```python
from build123d import *

# Parameters (mm, degrees)
F1_DEPTH = 190
F0_W     = 80
F0_H     = 30.028
F0_W_2   = 35.56
F0_H_2   = 17.78
F0_H_3   = 9.652
F0_W_3   = 2.22
F2_DEPTH = 5


with BuildPart() as f1:
    # F0 (on Front) → F1 (new body)
    with BuildSketch(Plane.XZ):
        Polygon((45, 30), (45, 35), (-40, 35), (-40, 30.452), (-40, 30), (40, 30), align=None)
        Polygon((-40, 30.452), (-40, 35), (-45, 35), (-45, -30), (-40, -30), (-40, -20.348), (-40, -19.078), (-40, -1.298), (-40, -0.028), (-40, 30), align=None)
        Polygon((45, -30), (45, 30), (40, 30), (40, -0.028), (40, -1.298), (40, -19.078), (40, -20.348), (40, -30), align=None)
        Polygon((45, -35), (45, -30), (40, -30), (4.44, -30), (2.22, -30), (-2.22, -30), (-4.44, -30), (-40, -30), (-45, -30), (-45, -35), align=None)
        Polygon((40, -1.298), (40, -0.028), (-40, -0.028), (-40, -1.298), (-4.44, -1.298), (-2.22, -1.298), (2.22, -1.298), (4.44, -1.298), align=None)
        Polygon((4.44, -20.348), (40, -20.348), (40, -19.078), (4.44, -19.078), (2.22, -19.078), (2.22, -20.348), align=None)
        Polygon((-40, -19.078), (-40, -20.348), (-4.44, -20.348), (-2.22, -20.348), (-2.22, -19.078), (-4.44, -19.078), align=None)
        Polygon((-2.22, -30), (2.22, -30), (2.22, -20.348), (2.22, -19.078), (2.22, -1.298), (-2.22, -1.298), (-2.22, -19.078), (-2.22, -20.348), align=None)
    extrude(amount=F1_DEPTH)

    # F0 (on Front) → F2 (join)
    with BuildSketch(Plane.XZ):
        with Locations((0, 14.986)):
            Rectangle(F0_W, F0_H)
        with Locations((-22.22, -10.188)):
            Rectangle(F0_W_2, F0_H_2)
        with Locations((22.22, -10.188)):
            Rectangle(F0_W_2, F0_H_2)
        with Locations((22.22, -25.174)):
            Rectangle(F0_W_2, F0_H_3)
        with Locations((-22.22, -25.174)):
            Rectangle(F0_W_2, F0_H_3)
        with Locations((-3.33, -10.188)):
            Rectangle(F0_W_3, F0_H_2)
        with Locations((-3.33, -25.174)):
            Rectangle(F0_W_3, F0_H_3)
        with Locations((3.33, -25.174)):
            Rectangle(F0_W_3, F0_H_3)
        with Locations((3.33, -10.188)):
            Rectangle(F0_W_3, F0_H_2)
    extrude(amount=F2_DEPTH)


solid = f1.part
```
Geometry: final body of the model. Coordinates: model frame, mm. A direction names the side the tool comes from. Round coordinates to 2 decimals unless told otherwise and drop trailing zeros. Write each loop counter-clockwise with the first axis right and the second up, starting at its lowest first coordinate (ties: lowest second). Pieces come first, ordered by that corner, then holes. Notation, with made-up numbers: (-17, 30.25) -> (38, 30.25) arc R21 cw to (38, 69.25) -> close; hole circle Ø2 at (70.5, 70). An arc over 180 degrees is marked (long way). Return JSON: item names as keys, results as strings.
Q1. Section A-A on x = 29.5. Return the cut outline in (y, z).
From the geometry:
{"outline": "(-190, -35) -> (0, -35) -> (0, 35) -> (-190, 35) -> (-190, 30) -> (-5, 30) -> (-5, -0.03) -> (-190, -0.03) -> (-190, -1.3) -> (-5, -1.3) -> (-5, -19.08) -> (-190, -19.08) -> (-190, -20.35) -> (-5, -20.35) -> (-5, -30) -> (-190, -30) -> close"}
Q2. First-contact query: pin 1 Ø5 at (x, z) = (-5.5, 15) entering from -Y. Flat tip, straight axial feed; report the tip coordinate or a pass-through.
From the geometry:
{"pin 1": "y = -5"}
Q3. Set-up query: faces 4 (the flat face through (-40, -96, 15)), 5 (the flat face through (0, -190, -5)). Return all of +Z, -Z, +X, -X, +Y, -Y with unobstructed straight access to the full face (end or side cutting, diameter ignored); none if empty.
From the geometry:
{"face 4": "-Y", "face 5": "+Z, -Z, +X, -X, -Y"}
Q4. Section B-B on z = 6. Return the cut outline in (x, y).
From the geometry:
{"outline": "(-45, -190) -> (-40, -190) -> (-40, -5) -> (40, -5) -> (40, -190) -> (45, -190) -> (45, 0) -> (-45, 0) -> close"}
Q5. Section D-D on z = -6. Return the cut outline in (x, y), and give its area (3 significant figures).
From the geometry:
{"outline": "(-45, -190) -> (-40, -190) -> (-40, -5) -> (-2.22, -5) -> (-2.22, -190) -> (2.22, -190) -> (2.22, -5) -> (40, -5) -> (40, -190) -> (45, -190) -> (45, 0) -> (-45, 0) -> close", "area": "3,120 mm2"}
Q6. Ray query, line 1 (Z direction, x = 36, y = -124); line 2 (X direction, y = -111, z = -18); line 3 (X direction, y = -97.5, z = 18.5). Return the intervals inside material, ascending.
From the geometry:
{"line 1": "-35 to -30, -20.35 to -19.08, -1.3 to -0.03, 30 to 35", "line 2": "-45 to -40, -2.22 to 2.22, 40 to 45", "line 3": "-45 to -40, 40 to 45"}
Q7. Section C-C on y = -147. Return the cut outline in (x, z), and give its area (4 significant figures).
From the geometry:
{"outline": "(-45, -35) -> (45, -35) -> (45, 35) -> (-45, 35) -> close; hole (-40, -30) -> (-2.22, -30) -> (-2.22, -20.35) -> (-40, -20.35) -> close; hole (-40, -19.08) -> (-2.22, -19.08) -> (-2.22, -1.3) -> (-40, -1.3) -> close; hole (-40, -0.03) -> (40, -0.03) -> (40, 30) -> (-40, 30) -> close; hole (2.22, -30) -> (40, -30) -> (40, -20.35) -> (2.22, -20.35) -> close; hole (2.22, -19.08) -> (40, -19.08) -> (40, -1.3) -> (2.22, -1.3) -> close", "area": "1,825 mm2"}
Q8. Mould query, pull axis X, two halves, no side actions, for faces 1 (the flat face through (-45, -94, 0)), 2 (the flat face through (1, -96, -0.028)), 3 (the flat face through (1, -94, 35)). Classes: +X half, -X half, draft (parallel to the pull), parting line (faces both ways), or undercut.
From the geometry:
{"face 1": "-X half", "face 2": "undercut", "face 3": "draft"}
